Input: part model. Units: mm. Frame: model coordinates. A direction names the side the tool comes from. Coordinates: 2 decimals unless noted, no trailing zeros. Loops run counter-clockwise (first coordinate to the right, second up) from the corner with the lowest first, then second, coordinate; pieces in that order, holes last.
```python
from build123d import *

# Parameters (mm, degrees)
SKETCH_W        = 48.55
SKETCH_H        = 24.45
PAD_DEPTH       = 4.9
SKETCH001_W     = 45.55
SKETCH001_H     = 20.45
POCKET_DEPTH    = 1.6
SKETCH002_R     = 8.08
POCKET001_DEPTH = 3.3
SKETCH003_W     = 10.65
SKETCH003_H     = 2.8
POCKET002_DEPTH = 1.6


with BuildPart() as part:
    # Sketch → Pad (new body)
    with BuildSketch(Plane.XY):
        with Locations((24.275, 12.225)):
            Rectangle(SKETCH_W, SKETCH_H)
    extrude(amount=PAD_DEPTH)

    # Sketch001 → Pocket (cut)
    with BuildSketch(Plane.XY.offset(4.9)):
        with Locations((24.275, 11.725)):
            Rectangle(SKETCH001_W, SKETCH001_H)
    extrude(amount=-POCKET_DEPTH, mode=Mode.SUBTRACT)

    # Sketch002 → Pocket001 (cut)
    with BuildSketch(Plane.XY.offset(3.3)):
        with Locations((11.0875, 11.7175)):
            Circle(SKETCH002_R)
        with Locations((37.4625, 11.7175)):
            Circle(SKETCH002_R)
        with BuildLine():
            Line((20.624978, 21.62), (27.924978, 21.62))
            ThreePointArc((27.925, 16.68), (30.394994, 19.150011), (27.924978, 21.62))
            Line((20.625, 16.68), (27.925, 16.68))
            ThreePointArc((20.624978, 21.62), (18.154979, 19.149989), (20.625, 16.68))
        make_face()
    extrude(amount=-POCKET001_DEPTH, mode=Mode.SUBTRACT)

    # Sketch003 → Pocket002 (cut)
    with BuildSketch(Plane.XY.offset(3.3)):
        with Locations((24.275, 2.9)):
            Rectangle(SKETCH003_W, SKETCH003_H)
    extrude(amount=-POCKET002_DEPTH, mode=Mode.SUBTRACT)


solid = part.part
```
Item 1: Section query C-C (y = 18.25). Output: boundary loops of the cut face in (x, z), then the cut area to 3 significant figures.
Result:
outline: (0, 0) - (6.33, 0) - (6.33, 3.3) - (1.5, 3.3) - (1.5, 4.9) - (0, 4.9) - close; (15.84, 0) - (18.32, 0) - (18.32, 3.3) - (15.84, 3.3) - close; (30.23, 0) - (32.71, 0) - (32.71, 3.3) - (30.23, 3.3) - close; (42.22, 0) - (48.55, 0) - (48.55, 4.9) - (47.05, 4.9) - (47.05, 3.3) - (42.22, 3.3) - close
area: 63.0 mm2
Item 2: Contact query for flat-ended pins moving along their axis: P1, Ø0.5, axis at x = 22.5, z = 3, coming from the -Y side; P2, Ø1.4, axis at x = 23.5, y = 3.5, coming from the +Z side; P3, Ø10, axis at x = 34.5, y = 7.5, coming from the +Z side. Output: stop coordinate, or through.
Result:
P1: stops at y = 0
P2: stops at z = 1.7
P3: stops at z = 3.3
Item 3: Section query B-B (x = 37). Output: boundary loops of the cut face in (y, z).
Result:
outline: (0, 0) - (3.65, 0) - (3.65, 3.3) - (1.5, 3.3) - (1.5, 4.9) - (0, 4.9) - close; (19.78, 0) - (24.45, 0) - (24.45, 4.9) - (21.95, 4.9) - (21.95, 3.3) - (19.78, 3.3) - close
Item 4: Mould query, pull axis Y, two halves, no side actions, for faces 1 (the face through (48.55, 12, 2)), 2 (the face through (24, 0, 2)), 3 (the face through (18.156, 19.204, 1.673)). Classes: +Y half, -Y half, draft (parallel to the pull), parting line (faces both ways), or undercut.
Result:
face 1: draft
face 2: -Y half
face 3: undercut
Item 5: Reachability of faces 4 (the face through (0, 12, 2)), 5 (the face through (29.6, 3, 3)), 6 (the face through (24, 21.62, 2)) from +Z, -Z, +X, -X, +Y, -Y: full face, straight path, thin tool, end or side. Return the list, or none.
Result:
face 4: +Z, -Z, -X, +Y, -Y
face 5: +Z
face 6: +Z, -Z
Item 6: Section query A-A (z = 3.85). Output: boundary loops of the cut face in (x, y).
Result:
outline: (0, 0) - (48.55, 0) - (48.55, 24.45) - (0, 24.45) - close; hole (1.5, 1.5) - (47.05, 1.5) - (47.05, 21.95) - (1.5, 21.95) - close
Item 7: Section query D-D (y = 20.75). Output: boundary loops of the cut face in (x, z), then the cut area to 3 significant figures.
Result:
outline: (0, 0) - (18.74, 0) - (18.74, 3.3) - (1.5, 3.3) - (1.5, 4.9) - (0, 4.9) - close; (29.81, 0) - (48.55, 0) - (48.55, 4.9) - (47.05, 4.9) - (47.05, 3.3) - (29.81, 3.3) - close
area: 129 mm2
Item 8: Line query: L1, parallel to X at y = 18.75, z = 3.85; L2, parallel to Y at x = 24.5, z = 3.6; L3, parallel to Y at x = 26.5, z = 0.3. Output: solid intervals per line, ascending.
Result:
L1: x = 0 to 1.5, 47.05 to 48.55
L2: y = 0 to 1.5, 21.95 to 24.45
L3: y = 0 to 16.68, 21.62 to 24.45
